For this review, take the finished solid that the model builds, in its own axes (mm). Face numbers are marked on the shaded views. A direction names the side the tool comes from. Give positions to 0.01 mm unless a question says otherwise; leave off trailing zeros. One line per item, written item: value. Start each with the question number.
Item 1: To check wall thickness, follow probe 1 along Z at (x, y) = (-5.75, 227.1); probe 2 along X at (y, z) = (226.4, -149); probe 3 along Y at (x, z) = (-11.25, -150.15). State the ranges of each line that lie inside material, in increasing order.
Item 2: Clearance check with flat-ended pins moving along their axes: pin 1 Ø3 at (y, z) = (228.5, -152.5) entering from -X; pin 2 Ø1.5 at (y, z) = (228, -150.5) entering from -X; pin 3 Ø2 at (x, y) = (-2, 228) entering from +Z; pin 4 Ø1 at (x, y) = (-12.5, 225.5) entering from +Z. State where each tip first meets the part, or that it passes through.
Item 3: Consider section A-A, the plane x = -9. Give the number of separate pieces and of enclosed holes in the cut face, and give its area (3 significant figures).
Item 4: Tool access review of the marked faces 1 and 2: name each direction out of +Z, -Z, +X, -X, +Y, -Y from which nothing blocks a thin tool from reaching the whole face with its end or side.
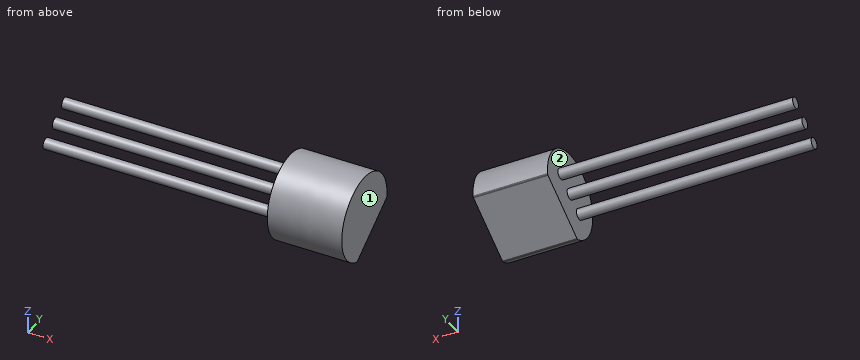
```python
from build123d import *

# Parameters (mm, degrees)
BOSS_EXTRUDE1_DEPTH = 4.6
BOSS_EXTRUDE2_DEPTH = 14.5


with BuildPart() as part:
    # Sketch1 → Boss-Extrude1 (new body)
    with BuildSketch(Plane.YZ):
        with BuildLine():
            Line((229.674293499, -151.143340678), (226.326149061, -153.290122953))
            Line((226.326149061, -153.290122953), (226.272491625, -153.307881389))
            Line((226.272491625, -153.307881389), (226.216442541, -153.300599253))
            add(Edge.make_bspline(
                [(226.216442541, -153.300599253), (225.874904083, -153.174533582), (225.580435107, -152.959521565), (225.286628269, -152.74499302), (225.062097982, -152.457360168), (224.838244561, -152.170594409), (224.701034241, -151.832482244), (224.564237553, -151.495389348), (224.52483063, -151.132631023), (224.485542502, -150.770966265), (224.546949824, -150.411277999), (224.608172029, -150.052674045), (224.765701828, -149.723537492), (224.92275674, -149.39539315), (225.164373094, -149.121955689), (225.405261075, -148.849342529), (225.712503507, -148.652495899), (226.01881973, -148.45624268), (226.368213662, -148.351026769), (226.716554316, -148.24612804), (227.081404623, -148.240581773), (227.445155058, -148.235052226), (227.797585685, -148.329599361), (228.14895388, -148.423861475), (228.462037686, -148.611278225), (228.774177674, -148.79812999), (229.023993777, -149.064096948), (229.273056788, -149.329262125), (229.440518215, -149.653458328), (229.607474816, -149.976677214), (229.67978683, -150.334332747), (229.751936455, -150.691185103), (229.723518522, -151.054698615)],
                knots=[0, 0, 0, 0.0625, 0.0625, 0.125, 0.125, 0.1875, 0.1875, 0.25, 0.25, 0.3125, 0.3125, 0.375, 0.375, 0.4375, 0.4375, 0.5, 0.5, 0.5625, 0.5625, 0.625, 0.625, 0.6875, 0.6875, 0.75, 0.75, 0.8125, 0.8125, 0.875, 0.875, 0.9375, 0.9375, 1, 1, 1], degree=2))
            Line((229.723518522, -151.054698615), (229.706686704, -151.108654203))
            Line((229.706686704, -151.108654203), (229.674293499, -151.143340678))
        make_face()
    extrude(amount=BOSS_EXTRUDE1_DEPTH)

    # Sketch2 → Boss-Extrude2 (add)
    with BuildSketch(Plane(origin=(0, 0, 0), x_dir=(0, -1, 0), z_dir=(-1, 0, 0))):
        with BuildLine():
            add(Edge.make_bspline(
                [(-225.765572547, -151.715949147), (-225.741758397, -151.67876225), (-225.708923966, -151.594914599), (-225.711552038, -151.459869117), (-225.765659729, -151.33610908), (-225.863009632, -151.242475831), (-225.988781109, -151.193224184), (-226.123826591, -151.195852256), (-226.247586628, -151.249959946), (-226.341219877, -151.34730985), (-226.390471524, -151.473081327), (-226.387843452, -151.608126809), (-226.333735761, -151.731886846), (-226.236385858, -151.825520095), (-226.110614381, -151.874771742), (-225.975568899, -151.87214367), (-225.851808862, -151.818035979), (-225.789386696, -151.753136043), (-225.765572547, -151.715949147)],
                knots=[0, 0, 0, 0, 0.0625, 0.125, 0.1875, 0.25, 0.3125, 0.375, 0.4375, 0.5, 0.5625, 0.625, 0.6875, 0.75, 0.8125, 0.875, 0.9375, 1, 1, 1, 1], degree=3))
        make_face()
        with BuildLine():
            add(Edge.make_bspline(
                [(-226.835067383, -151.031054414), (-226.811253234, -150.993867518), (-226.778418803, -150.910019867), (-226.781046875, -150.774974384), (-226.835154565, -150.651214347), (-226.932504469, -150.557581098), (-227.058275945, -150.508329452), (-227.193321428, -150.510957524), (-227.317081465, -150.565065214), (-227.410714714, -150.662415118), (-227.45996636, -150.788186594), (-227.457338289, -150.923232076), (-227.403230598, -151.046992114), (-227.305880694, -151.140625362), (-227.180109218, -151.189877009), (-227.045063736, -151.187248937), (-226.921303698, -151.133141247), (-226.858881533, -151.068241311), (-226.835067383, -151.031054414)],
                knots=[0, 0, 0, 0, 0.0625, 0.125, 0.1875, 0.25, 0.3125, 0.375, 0.4375, 0.5, 0.5625, 0.625, 0.6875, 0.75, 0.8125, 0.875, 0.9375, 1, 1, 1, 1], degree=3))
        make_face()
        with BuildLine():
            add(Edge.make_bspline(
                [(-227.90456222, -150.346159682), (-227.880748071, -150.308972785), (-227.847913639, -150.225125134), (-227.850541711, -150.090079652), (-227.904649402, -149.966319615), (-228.001999305, -149.872686366), (-228.127770782, -149.823434719), (-228.262816264, -149.826062791), (-228.386576301, -149.880170482), (-228.48020955, -149.977520385), (-228.529461197, -150.103291862), (-228.526833125, -150.238337344), (-228.472725435, -150.362097381), (-228.375375531, -150.45573063), (-228.249604054, -150.504982277), (-228.114558572, -150.502354205), (-227.990798535, -150.448246514), (-227.928376369, -150.383346579), (-227.90456222, -150.346159682)],
                knots=[0, 0, 0, 0, 0.0625, 0.125, 0.1875, 0.25, 0.3125, 0.375, 0.4375, 0.5, 0.5625, 0.625, 0.6875, 0.75, 0.8125, 0.875, 0.9375, 1, 1, 1, 1], degree=3))
        make_face()
    extrude(amount=BOSS_EXTRUDE2_DEPTH)


solid = part.part
```
Model answer:
1. probe 1: z = -151.19 to -150.51
1. probe 2: x = 0 to 4.6
1. probe 3: y = 227.85 to 228.53
2. pin 1: stops at x = 0
2. pin 2: stops at x = -14.5
2. pin 3: stops at z = -149.83
2. pin 4: stops at z = -151.2
3. separate pieces: 3
3. enclosed holes: 0
3. area: 1.07 mm2
4. face 1: +Z, -Z, +X, +Y, -Y
4. face 2: -X
